Part model, mm, in its own coordinate system. Give positions to 0.01 mm unless a question says otherwise; leave off trailing zeros. Order: outer loops, then holes, each group sorted by start corner. A loop starts at its lowest first (then second) coordinate and runs counter-clockwise, first axis right, second up.
1. Probe line 1 (X direction, y = 2.75, z = 0); line 2 (X direction, y = 4.5, z = 13.5); line 3 (Z direction, x = 30, y = 3). List the from-to ranges inside material, lowest first.
2. Slice it at B-B on z = 0. List the corners of the cut face in (x, y).
3. Slice it at A-A on x = 0. List the corners of the cut face in (y, z), and give its area (3 significant figures).
4. Drop flat-ended pins along their axis: pin 1 Ø4 at (x, y) = (19, -4.5) entering from -Z; pin 2 Ø6 at (y, z) = (3, 14.5) entering from +X; pin 3 Ø3 at (y, z) = (2.5, -57.5) entering from -X. Give the stop position or say it passes through.
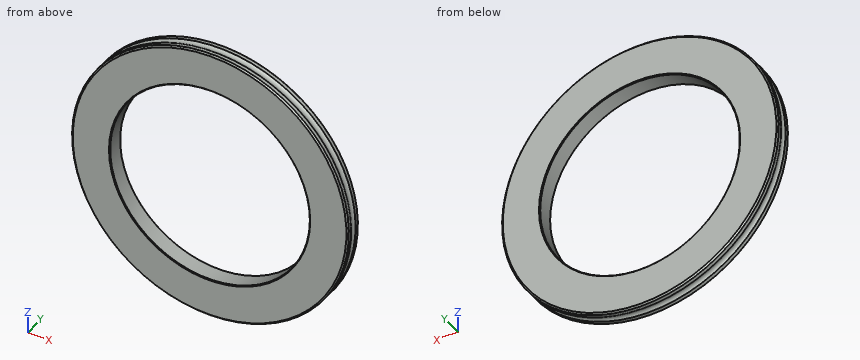
from build123d import *

# Parameters (mm, degrees)
HOLE_WIZARD_2_D = 133.5
CHAMFER_1_SIZE  = 0.5
CHAMFER_2_SIZE2 = 1.000000001
CHAMFER_2_SIZE  = 0.999999999


with BuildPart() as part:
    # 草圖1 → 旋轉1 (revolve)
    with BuildSketch(Plane.XY, mode=Mode.PRIVATE) as revolve_1_sk:
        with BuildLine():
            Line((92.5, 6), (0, 6))
            Line((0, 6), (0, -6))
            Line((0, -6), (92.5, -6))
            Line((92.5, -6), (92.5, -2.449489743))
            ThreePointArc((92.5, -2.449489743), (91.5, 0), (92.5, 2.449489743))
            Line((92.5, 2.449489743), (92.5, 6))
        make_face()
    revolve(revolve_1_sk.sketch.rotate(Axis((0, 6, 0), (0, -1, 0)), 270), axis=Axis((0, 6, 0), (0, -1, 0)))

    # 鑽孔2 (through all)
    with Locations(Plane(origin=(0, -6, 0), x_dir=(-1, 0, 0), z_dir=(0, -1, 0))):
        with Locations((0, 0)):
            Hole(HOLE_WIZARD_2_D / 2)

    # 導角1
    chamfer_1_edges = [part.edges().sort_by_distance(p)[0] for p in [
        (-66.75, -6, 0),
        (-66.75, 6, 0),
    ]]
    chamfer(chamfer_1_edges, length=CHAMFER_1_SIZE)

    # 導角2
    chamfer_2_edges = [part.edges().sort_by_distance(p)[0] for p in [
        (0, 6, 92.5),
        (0, -6, 92.5),
    ]]
    chamfer(chamfer_2_edges, length=CHAMFER_2_SIZE, length2=CHAMFER_2_SIZE2)


solid = part.part
Data:
1. line 1: x = -92.5 to -66.75, 66.75 to 92.5
1. line 2: x = -91.51 to -65.37, 65.37 to 91.51
1. line 3: z = -87.5 to -59.63, 59.63 to 87.5
2. outline: (-92.5, -5) - (-91.5, -6) - (-67.25, -6) - (-66.75, -5.5) - (-66.75, 5.5) - (-67.25, 6) - (-91.5, 6) - (-92.5, 5) - (-92.5, 2.45) arc R3.5 cw to (-92.5, -2.45) - close; (66.75, -5.5) - (67.25, -6) - (91.5, -6) - (92.5, -5) - (92.5, -2.45) arc R3.5 cw to (92.5, 2.45) - (92.5, 5) - (91.5, 6) - (67.25, 6) - (66.75, 5.5) - close
3. outline: (-6, -91.5) - (-5, -92.5) - (-2.45, -92.5) arc R3.5 cw to (2.45, -92.5) - (5, -92.5) - (6, -91.5) - (6, -67.25) - (5.5, -66.75) - (-5.5, -66.75) - (-6, -67.25) - close; (-6, 67.25) - (-5.5, 66.75) - (5.5, 66.75) - (6, 67.25) - (6, 91.5) - (5, 92.5) - (2.45, 92.5) arc R3.5 cw to (-2.45, 92.5) - (-5, 92.5) - (-6, 91.5) - close
3. area: 609 mm2
4. pin 1: stops at z = -90.92
4. pin 2: stops at x = 91.78
4. pin 3: stops at x = -73.62
